from build123d import *

# Parameters (mm, degrees)
SK_PLACA_TOPE_R   = 5.1
SK_PLACA_TOPE_R_2 = 0.75
PLACA_TOPE_DEPTH  = 2


with BuildPart() as part:
    # Sk_Placa_tope → Placa_tope (new body)
    with BuildSketch(Plane.XY.offset(52.4)):
        with BuildLine():
            Line((-8.014047084, -36.814047084), (3.450714432, -38.949285568))
            ThreePointArc((3.450714432, -38.949285568), (6.121320344, -38.121320344), (6.949285568, -35.450714432))
            Line((6.949285568, -35.450714432), (4.814047084, -23.985952916))
            ThreePointArc((4.814047084, -23.985952916), (-13.778174593, -18.221825407), (-8.014047084, -36.814047084))
        make_face()
        with Locations((-6, -26)):
            Circle(SK_PLACA_TOPE_R, mode=Mode.SUBTRACT)
        with Locations((-1, -20)):
            Circle(SK_PLACA_TOPE_R_2, mode=Mode.SUBTRACT)
        with Locations((1.5, -24)):
            Circle(SK_PLACA_TOPE_R_2, mode=Mode.SUBTRACT)
    extrude(amount=PLACA_TOPE_DEPTH)


solid = part.part
The listing builds one solid part. Answer for the finished solid, in the listing's coordinates (mm). Coordinates: 2 decimals unless noted, no trailing zeros. Write each loop counter-clockwise with the first axis right and the second up, starting at its lowest first coordinate (ties: lowest second). Pieces come first, ordered by that corner, then holes. Notation, with made-up numbers: M 35,37.25 L 67,37.25 A4 cw 67,41.25 Z; hole C 78.5,57.25 d7. An arc over 180 degrees is marked long. Put each result on its own line as item: value. Start each with the question number.
1. A cutting plane is placed at D-D on x = -12. Write down the section's boundary in (y, z), then the cut area to 3 significant figures.
2. For a pull along X with two mould halves and no side action, classify faces 1 (the cylindrical face through (-1.163, -20.732, 53.386)), 2 (the cylindrical face through (1.337, -24.732, 53.386)), 3 (the flat face through (-5, -32, 54.4)), 4 (the flat face through (5.897, -29.799, 53.386)) as pulls with the +X half, pulls with the -X half, needs draft (parallel to the pull), parting line crosses it, or undercut.
3. A cutting plane is placed at B-B on y = -26. Write down the section's boundary in (x, z).
4. Consider line 1 (X direction, y = -23.75, z = 53); line 2 (X direction, y = -21.5, z = 53.9); line 3 (Y direction, x = -7.75, z = 54.2). Determine where each line is inside the solid, lowest interval first. Write a range as from..to.
5. A cutting plane is placed at A-A on z = 53. Write down the section's boundary in (x, y).
6. A cutting plane is placed at C-C on x = -6. Write down the section's boundary in (y, z).
7. Flat-ended cylindrical pins translate along their axes: P1, Ø1, axis at y = -30.5, z = 52.5, coming from the +X side; P2, Ø1, axis at x = 0, z = 53.5, coming from the -Y side. Find the tip coordinate at first contact, or state that the pin passes through.
Resolved:
1. outline: M -35.22,52.4 L -16.78,52.4 L -16.78,54.4 L -35.22,54.4 Z
1. area: 36.9 mm2
2. face 1: undercut
2. face 2: undercut
2. face 3: needs draft
2. face 4: pulls with the +X half
3. outline: M -17,52.4 L -11.1,52.4 L -11.1,54.4 L -17,54.4 Z; M -0.9,52.4 L 5.19,52.4 L 5.19,54.4 L -0.9,54.4 Z
4. line 1: x = -16.77..-10.58, -1.42..0.79, 2.21..4.77
4. line 2: x = -16.04..-8.4, -3.6..4.04
4. line 3: y = -36.86..-30.79, -21.21..-15.14
5. outline: M -8.01,-36.81 L 3.45,-38.95 A3 ccw 6.95,-35.45 L 4.81,-23.99 A11 ccw long Z; hole C -6,-26 d10.2; hole C -1,-20 d1.5; hole C 1.5,-24 d1.5
6. outline: M -37.19,52.4 L -31.1,52.4 L -31.1,54.4 L -37.19,54.4 Z; M -20.9,52.4 L -15,52.4 L -15,54.4 L -20.9,54.4 Z
7. P1: stops at x = 6.12
7. P2: stops at y = -38.4
